Source: CAD feature listing. Evaluate the final solid. Frame: model axes, mm. A direction names the side the tool comes from. Round coordinates to 2 decimals unless told otherwise and drop trailing zeros. Loops run counter-clockwise (first coordinate to the right, second up) from the corner with the lowest first, then second, coordinate; pieces in that order, holes last. Notation, with made-up numbers: M 48.5,87.25 L 70.5,87.25 A15 ccw 70.5,105.25 Z; hole C 38,-25 d5. An arc over 180 degrees is marked long. One line per item, written item: value.
from build123d import *

# Parameters (mm, degrees)
F0_R     = 7
F1_DEPTH = 105
F2_R     = 11.7037675531
F2_R_2   = 7
F3_DEPTH = 25
F4_R     = 5
F6_DEPTH = 20
F7_DEPTH = 3


with BuildPart() as f1:
    # F0 (on Top) → F1 (new body)
    with BuildSketch(Plane.XY):
        with Locations((-4.6541057527, 0)):
            Circle(F0_R)
    extrude(amount=F1_DEPTH)

    # F2 (on face) → F3 (join)
    with BuildSketch(Plane(origin=(0, 0, 0), x_dir=(1, 0, 0), z_dir=(0, 0, -1))):
        with Locations((-4.6541057527, 0)):
            Circle(F2_R)
        with Locations((-4.6541057527, 0)):
            Circle(F2_R_2, mode=Mode.SUBTRACT)
        with Locations((-4.6541057527, 0)):
            Circle(F2_R_2)
    extrude(amount=F3_DEPTH)

    # F4
    f4_edges = [f1.edges().sort_by_distance(p)[0] for p in [
        (-16.357873, 0, -25),
    ]]
    fillet(f4_edges, radius=F4_R)

    # F5 (on face) → F6 (cut)
    with BuildSketch(Plane.XY):
        with BuildLine():
            Line((-12.4576410745, 8.2758134023), (-4.6541057527, 11.7037675531))
            ThreePointArc((-4.6541057527, 11.7037675531), (-9.1329436915, 10.8128712956), (-12.929919155, 8.2758134023))
            Line((-12.929919155, 8.2758134023), (-12.4576410745, 8.2758134023))
        make_face()
        with BuildLine():
            ThreePointArc((-12.929919155, 8.2758134023), (-15.4669770483, 4.4788379388), (-16.3578733058, 0))
            Line((-16.3578733058, 0), (-12.929919155, 7.727174844))
            Line((-12.929919155, 7.727174844), (-12.929919155, 8.2758134023))
        make_face()
        with BuildLine():
            ThreePointArc((3.6217076495, 8.2758134023), (-0.1752678139, 10.8128712956), (-4.6541057527, 11.7037675531))
            Line((-4.6541057527, 11.7037675531), (3.6217076495, 8.2758134023))
        make_face()
        with BuildLine():
            Line((3.6217076495, 8.2758134023), (7.0496618004, 0))
            ThreePointArc((7.0496618004, 0), (6.1587655429, 4.4788379388), (3.6217076495, 8.2758134023))
        make_face()
        with BuildLine():
            ThreePointArc((3.6217076495, -8.2758134023), (6.1587655429, -4.4788379388), (7.0496618004, 0))
            Line((7.0496618004, 0), (3.6217076495, -8.2758134023))
        make_face()
        with BuildLine():
            Line((3.6217076495, -8.2758134023), (-4.6541057527, -11.7037675531))
            ThreePointArc((-4.6541057527, -11.7037675531), (-0.1752678139, -10.8128712956), (3.6217076495, -8.2758134023))
        make_face()
        with BuildLine():
            Line((-12.929919155, -8.2758134023), (-16.3578733058, 0))
            ThreePointArc((-16.3578733058, 0), (-15.4669770483, -4.4788379388), (-12.929919155, -8.2758134023))
        make_face()
        with BuildLine():
            ThreePointArc((-12.929919155, -8.2758134023), (-9.1329436915, -10.8128712956), (-4.6541057527, -11.7037675531))
            Line((-4.6541057527, -11.7037675531), (-12.929919155, -8.2758134023))
        make_face()
    extrude(amount=-F6_DEPTH, mode=Mode.SUBTRACT)

    # F7 (cut): a face of the model
    f7_faces = [f1.faces().sort_by_distance(p)[0] for p in [
        (-4.6541057527, 0, -25),
    ]]
    extrude(f7_faces, amount=-F7_DEPTH, mode=Mode.SUBTRACT)


solid = f1.part
1. Pin query (flat end, axial travel): pin 1 (4 mm diameter, centred on x = 4.5, y = -4, fed in from +Z); pin 2 (1.7 mm diameter, centred on x = 6, y = 5.5, fed in from +Z); pin 3 (8 mm diameter, centred on x = -1.5, z = -5, fed in from +Y). Return the tip coordinate at first contact, or that it passes through.
Report:
pin 1: stops at z = 0
pin 2: stops at z = -20
pin 3: stops at y = 11.7
2. Pull-direction query (Y, two-part tool) for faces 1 (the face through (6, 4, -20)), 2 (the face through (-5, 0, -22)), 3 (the face through (-14.62, -4.2, -9.86)); classes: released by +Y, released by -Y, zero draft, split by the parting line, or undercut.
Report:
face 1: zero draft
face 2: undercut
face 3: released by -Y
3. Section query A-A (z = 46). Return the cut outline in (x, y), and give its area (3 significant figures).
Report:
outline: C -4.65,0 d14
area: 154 mm2
4. Reachability of faces 4 (the face through (-0.57, 10.01, -9.86)), 5 (the face through (-9.974, 4.079, -23.521)), 6 (the face through (-15, 4, -20)), 7 (the face through (-15, -4, -20)) from +Z, -Z, +X, -X, +Y, -Y: full face, straight path, thin tool, end or side. Return the list, or none.
Report:
face 4: +Z, +X, +Y
face 5: -Z
face 6: +Z, -X, +Y
face 7: +Z, -X, -Y
5. Ray query, line 1 (Z direction, x = -5.25, y = -5.5); line 2 (X direction, y = 0, z = -23.35); line 3 (X direction, y = 0, z = -23.6). Return the intervals inside material, ascending. Write a range as [from, to].
Report:
line 1: z = [-22, 105]
line 2: x = [-15.07, -11.36], [2.05, 5.76]
line 3: x = [-14.83, -11.36], [2.05, 5.52]
